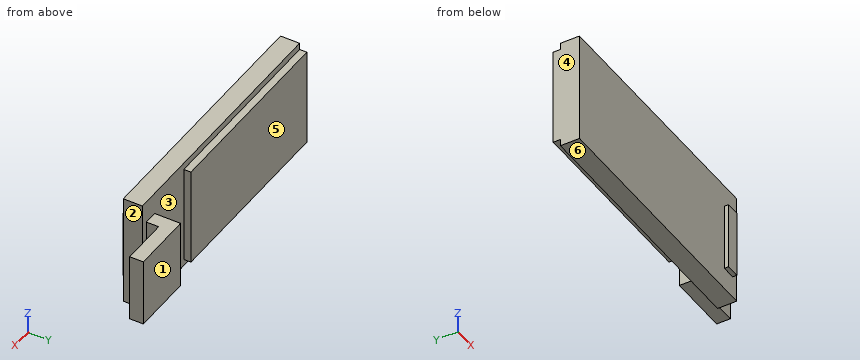
```python
from build123d import *

# Parameters (mm, degrees)
BOSS_EXTRUDE1_DEPTH      = 2.4
BOSS_EXTRUDE1_DEPTH_BACK = 0.4
SKETCH1_W                = 28
SKETCH1_H                = 14.5
BOSS_EXTRUDE2_START      = 2.4
SKETCH1_3_W              = 28
SKETCH1_3_H              = 14.5
BOSS_EXTRUDE2_DEPTH      = 1.05
BOSS_EXTRUDE3_DEPTH      = 5


with BuildPart() as part:
    # Sketch1 → Boss-Extrude1 (new, two sides: drawn at the far end of the back side and taken through both)
    with BuildSketch(Plane(origin=(0, 0, 0), x_dir=(1, 0, 0), z_dir=(0, 1, 0)).offset(-BOSS_EXTRUDE1_DEPTH_BACK)):
        Polygon((38, 8.25), (0, 8.25), (0, 7.25), (28, 7.25), (28, -7.25), (0, -7.25), (0, -8.25), (38, -8.25), align=None)
        with Locations((14, 0)):
            Rectangle(SKETCH1_W, SKETCH1_H)
    extrude(amount=BOSS_EXTRUDE1_DEPTH + BOSS_EXTRUDE1_DEPTH_BACK)

    # Sketch1<3> → Boss-Extrude2 (add)
    with BuildSketch(Plane(origin=(0, 0, 0), x_dir=(1, 0, 0), z_dir=(0, 1, 0)).offset(BOSS_EXTRUDE2_START)):
        with Locations((14, 0)):
            Rectangle(SKETCH1_3_W, SKETCH1_3_H)
    extrude(amount=BOSS_EXTRUDE2_DEPTH)

    # Sketch2 → Boss-Extrude3 (add, symmetric)
    with BuildSketch(Plane.XY):
        Polygon((37.032081111, -1), (35.032081111, -1), (35.032081111, 6.2), (44.032081111, 6.2), (44.032081111, 4.2), (37.032081111, 4.2), align=None)
    extrude(amount=BOSS_EXTRUDE3_DEPTH, both=True)


solid = part.part
```
For this review, take the finished solid that the model builds, in its own axes (mm). Face numbers are marked on the shaded views. A direction names the side the tool comes from. Give positions to 0.01 mm unless a question says otherwise; leave off trailing zeros. Order: outer loops, then holes, each group sorted by start corner. A loop starts at its lowest first (then second) coordinate and runs counter-clockwise, first axis right, second up.
1) Take a section at D-D (x = 20). Give the boundary of the cut face in (y, z).
2) Take a section at C-C (y = 5.75). Give the boundary of the cut face in (x, z), then the cut area to 3 significant figures.
3) Take a section at B-B (z = -1.75). Give the boundary of the cut face in (x, y).
4) Insertion check: pin 1 (0.8 mm diameter, centred on x = 18.5, y = 3, fed in from -Z); pin 2 (0.5 mm diameter, centred on y = 3, z = -1.5, fed in from +X); pin 3 (1.1 mm diameter, centred on x = 39, y = 4.5, fed in from +Z). Each pin has a flat end and moves straight along its axis. Give the tip position at first contact, or say it passes through.
5) Wall thickness on line 1 (Y direction, x = 37.5, z = -1.25); line 2 (Y direction, x = 31, z = 6.5); line 3 (X direction, y = 3, z = 6.5): over which ranges is each line inside the solid? List them lowest first.
6) The part is to be moulded in two halves that separate along X. For the marked faces 1, 2, 3 and 4, say which applies: released by +X, released by -X, zero draft, split by the parting line, or undercut.
7) Take a section at A-A (x = 35.5). Give the boundary of the cut face in (y, z).
8) For the marked faces 5 and 6, list the 3-axis set-ups (+Z, -Z, +X, -X, +Y, -Y) from which the entire face can be reached by the end or side of a thin tool; tool diameter is ignored.
Derived:
1. outline: (-0.4, -8.25) - (2.4, -8.25) - (2.4, -7.25) - (3.45, -7.25) - (3.45, 7.25) - (2.4, 7.25) - (2.4, 8.25) - (-0.4, 8.25) - close
2. outline: (35.03, -5) - (44.03, -5) - (44.03, 5) - (35.03, 5) - close
2. area: 90.0 mm2
3. outline: (0, -0.4) - (35.03, -0.4) - (35.03, -1) - (37.03, -1) - (37.03, -0.4) - (38, -0.4) - (38, 2.4) - (37.03, 2.4) - (37.03, 4.2) - (44.03, 4.2) - (44.03, 6.2) - (35.03, 6.2) - (35.03, 2.4) - (28, 2.4) - (28, 3.45) - (0, 3.45) - close
4. pin 1: stops at z = -7.25
4. pin 2: stops at x = 37.03
4. pin 3: stops at z = 5
5. line 1: y = -0.4 to 2.4, 4.2 to 6.2
5. line 2: y = -0.4 to 2.4
5. line 3: x = 0 to 28
6. face 1: zero draft
6. face 2: released by +X
6. face 3: undercut
6. face 4: released by -X
7. outline: (-1, -5) - (-0.4, -5) - (-0.4, -8.25) - (2.4, -8.25) - (2.4, -5) - (6.2, -5) - (6.2, 5) - (2.4, 5) - (2.4, 8.25) - (-0.4, 8.25) - (-0.4, 5) - (-1, 5) - close
8. face 5: +Z, -Z, -X, +Y
8. face 6: -Z, +X, -X, +Y, -Y
